Geometry check sheet. Reference: the model listing, model coordinates, mm. Round coordinates to 2 decimals unless told otherwise and drop trailing zeros. Loops run counter-clockwise (first coordinate to the right, second up) from the corner with the lowest first, then second, coordinate; pieces in that order, holes last. Notation, with made-up numbers: (-33.5, 80.25) - (-5.5, 80.25) arc R14 ccw to (-5.5, 106.25) - close; hole circle Ø8 at (-22, 78.25). An arc over 180 degrees is marked (long way). Write item = value, one per line.
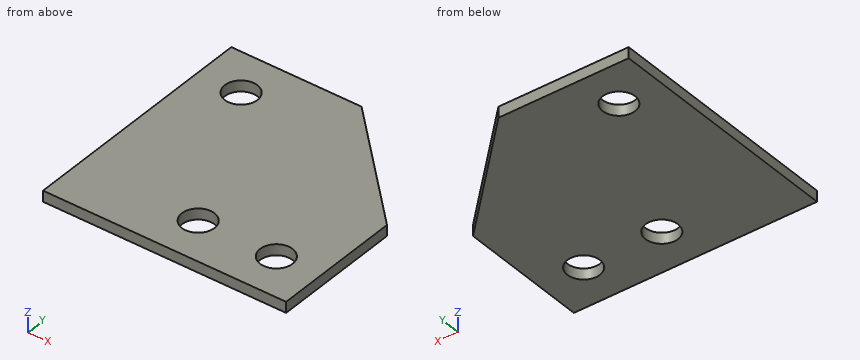
```python
from build123d import *

# Parameters (mm, degrees)
BOSS_EXTRUDE1_DEPTH            = 1.5875
F_3_16_0_1875_DIAMETER_HOLE1_D = 4.7625


with BuildPart() as part:
    # Sketch1 → Boss-Extrude1 (new body)
    with BuildSketch(Plane.XY):
        Polygon((19.05, 0), (35.56, -16.51), (35.56, -35.56), (0, -35.56), (0, 0), align=None)
    extrude(amount=BOSS_EXTRUDE1_DEPTH)

    # 3/16 (0.1875) Diameter Hole1 (through all)
    with Locations(Plane(origin=(0, 0, 0), x_dir=(-1, 0, 0), z_dir=(0, 0, -1))):
        with Locations((-6.35, -6.35), (-17.78, -29.21), (-29.21, -29.21)):
            Hole(F_3_16_0_1875_DIAMETER_HOLE1_D / 2)


solid = part.part
```
(1) Scan lines: L1, parallel to X at y = -30.5, z = 1; L2, parallel to X at y = -30, z = 0.65; L3, parallel to Y at x = 17.78, z = 0.7. Record each from-to range of solid material in increasing order. Write a range as [from, to].
Answers follow:
L1 = [0, 15.78], [19.78, 27.21], [31.21, 35.56]
L2 = [0, 15.53], [20.03, 26.96], [31.46, 35.56]
L3 = [-35.56, -31.59], [-26.83, 0]
(2) Section check B-B (y = -6.35). Enter the section's corners in (x, z).
Answers follow:
outline = (0, 0) - (3.97, 0) - (3.97, 1.59) - (0, 1.59) - close; (8.73, 0) - (25.4, 0) - (25.4, 1.59) - (8.73, 1.59) - close
(3) Section check D-D (y = -15). Enter the section's corners in (x, z), then the cut area to 3 significant figures.
Answers follow:
outline = (0, 0) - (34.05, 0) - (34.05, 1.59) - (0, 1.59) - close
area = 54.1 mm²
(4) Section check A-A (x = 29.21). Enter the section's corners in (y, z), then the cut area to 3 significant figures.
Answers follow:
outline = (-35.56, 0) - (-31.59, 0) - (-31.59, 1.59) - (-35.56, 1.59) - close; (-26.83, 0) - (-10.16, 0) - (-10.16, 1.59) - (-26.83, 1.59) - close
area = 32.8 mm²
(5) Section check C-C (z = 0.3). Enter the section's corners in (x, y).
Answers follow:
outline = (0, -35.56) - (35.56, -35.56) - (35.56, -16.51) - (19.05, 0) - (0, 0) - close; hole circle Ø4.76 at (6.35, -6.35); hole circle Ø4.76 at (17.78, -29.21); hole circle Ø4.76 at (29.21, -29.21)
(6) Gauge pin test, flat end, axial feed: pin 1 (7.5 mm diameter, centred on x = 6.35, y = -6.35, fed in from -Z). Record the tip position at first contact, or that the pin passes through.
Answers follow:
pin_1 = 0
